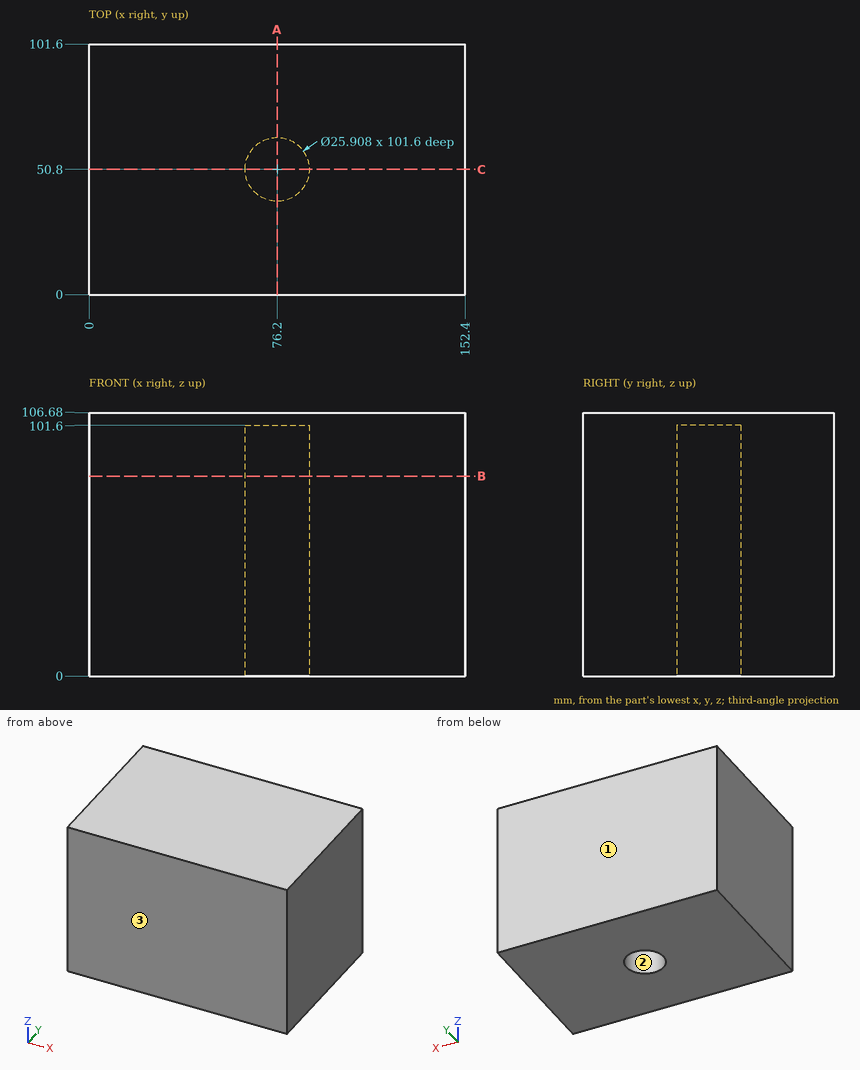
Answer from the drawing. Dimensions are ordinates in mm from the lowest x, y and z of the part. Round coordinates to 2 decimals unless told otherwise and drop trailing zeros. Loops run counter-clockwise (first coordinate to the right, second up) from the corner with the lowest first, then second, coordinate; pieces in that order, holes last. Notation, with made-up numbers: (15, 16.5) - (74, 16.5) arc R24 cw to (74, 55.5) - close; hole circle Ø3 at (-36, -34.5). An arc over 180 degrees is marked (long way). Return JSON: item names as keys, results as strings. Group by question number.
1. The part is cut by section B-B on z = 81. Determine the outline of the cut face in (x, y).
2. The part is cut by section C-C on y = 50.8. Determine the outline of the cut face in (x, z).
3. The part is cut by section A-A on x = 76.2. Determine the outline of the cut face in (y, z).
4. The mould has two halves that part along Y. Classify the marked faces 1, 2 and 3: pulls with the +Y half, pulls with the -Y half, needs draft (parallel to the pull), parting line crosses it, or undercut.
5. This flat-tipped pin is pushed along its axis until it touches: P1, Ø23.5, axis at x = 76.2, y = 50.8, coming from the -Z side. Where does it stop, or does it pass through?
6. Consider probe 1 along Y at (x, z) = (76, 48); probe 2 along X at (y, z) = (50, 39); probe 3 along Y at (x, z) = (72, 16). Determine where each line is inside the solid, lowest interval first.
Resolved:
{
 "1": {"outline": "(0, 0) - (152.4, 0) - (152.4, 101.6) - (0, 101.6) - close; hole circle Ø25.91 at (76.2, 50.8)"},
 "2": {"outline": "(0, 0) - (63.25, 0) - (63.25, 101.6) - (89.15, 101.6) - (89.15, 0) - (152.4, 0) - (152.4, 106.68) - (0, 106.68) - close"},
 "3": {"outline": "(0, 0) - (37.85, 0) - (37.85, 101.6) - (63.75, 101.6) - (63.75, 0) - (101.6, 0) - (101.6, 106.68) - (0, 106.68) - close"},
 "4": {"face 1": "pulls with the +Y half", "face 2": "undercut", "face 3": "pulls with the -Y half"},
 "5": {"P1": "stops at z = 101.6"},
 "6": {"probe 1": "y = 0 to 37.85, 63.75 to 101.6", "probe 2": "x = 0 to 63.27, 89.13 to 152.4", "probe 3": "y = 0 to 38.55, 63.05 to 101.6"}
}
